For this review, take the finished solid that the model builds, in its own axes (mm). A direction names the side the tool comes from. Give positions to 0.01 mm unless a question says otherwise; leave off trailing zeros. Write each loop counter-clockwise with the first axis right and the second up, starting at its lowest first coordinate (ties: lowest second). Pieces come first, ordered by that corner, then holes. Notation, with made-up numbers: (-24, 50.5) -> (-15, 50.5) arc R20 cw to (-15, 58.5) -> close; hole circle Ø7 at (89, 53.5). An arc over 180 degrees is marked (long way). Return JSON: item names as keys, results as strings.
Autodesk Fusion 360 part; units mm, degrees
sketch "Sketch1" plane through (0, 0, 0) normal (0, 0, 1) x (1, 0, 0)
  line L0 (36.9, -48.5) -> (-36.9, -48.5)
  line L1 (-36.9, -48.5) -> (-36.9, 48.5)
  line L2 (-36.9, 48.5) -> (36.9, 48.5)
  line L3 (36.9, 48.5) -> (36.9, -48.5)
  line L4 (36.9, -48.5) -> (-36.9, 48.5) construction
  line L5 (-36.9, -48.5) -> (36.9, 48.5) construction
  line L6 (35.35, -46.95) -> (-35.35, -46.95)
  line L7 (-35.35, -46.95) -> (-35.35, 46.95)
  line L8 (-35.35, 46.95) -> (35.35, 46.95)
  line L9 (35.35, 46.95) -> (35.35, -46.95)
  line L10 (35.35, -46.95) -> (-35.35, 46.95) construction
  line L11 (-35.35, -46.95) -> (35.35, 46.95) construction
  line L12 (35.35, -46.95) -> (0, -46.95)
  line L13 (0, -46.95) -> (0, -16.95)
  line L14 (11.5, -10.35) -> (-11.5, -10.35)
  line L15 (-11.5, -10.35) -> (-11.5, -23.55)
  line L16 (-11.5, -23.55) -> (11.5, -23.55)
  line L17 (11.5, -23.55) -> (11.5, -10.35)
  line L18 (11.5, -10.35) -> (-11.5, -23.55) construction
  line L19 (-11.5, -10.35) -> (11.5, -23.55) construction
  line L20 (13.775, -30.9) -> (-13.775, -30.9)
  line L21 (-13.775, -30.9) -> (-13.775, -3)
  line L22 (-13.775, -3) -> (13.775, -3)
  line L23 (13.775, -3) -> (13.775, -30.9)
  line L24 (13.775, -30.9) -> (-13.775, -3) construction
  line L25 (-13.775, -30.9) -> (13.775, -3) construction
  line L26 (13.775, -3) -> (11.975, -3)
  line L27 (-13.775, -3) -> (-11.975, -3)
  line L28 (-13.775, -30.9) -> (-11.975, -30.9)
  line L29 (13.775, -30.9) -> (11.975, -30.9)
  line L30 (-11.975, -30.9) -> (-13.775, -30.9)
  line L31 (-13.775, -30.9) -> (-13.775, -29.1)
  line L32 (-13.775, -29.1) -> (-11.975, -29.1)
  line L33 (-11.975, -29.1) -> (-11.975, -30.9)
  line L34 (11.975, -30.9) -> (13.775, -30.9)
  line L35 (13.775, -30.9) -> (13.775, -29.1)
  line L36 (13.775, -29.1) -> (11.975, -29.1)
  line L37 (11.975, -29.1) -> (11.975, -30.9)
  line L38 (-11.975, -3) -> (-13.775, -3)
  line L39 (-13.775, -3) -> (-13.775, -4.8)
  line L40 (-13.775, -4.8) -> (-11.975, -4.8)
  line L41 (-11.975, -4.8) -> (-11.975, -3)
  line L42 (11.975, -3) -> (13.775, -3)
  line L43 (13.775, -3) -> (13.775, -4.8)
  line L44 (13.775, -4.8) -> (11.975, -4.8)
  line L45 (11.975, -4.8) -> (11.975, -3)
  circle A0 centre (-11.975, -4.8) radius 1.1
  circle A1 centre (11.975, -4.8) radius 1.1
  circle A2 centre (11.975, -29.1) radius 1.1
  circle A3 centre (-11.975, -29.1) radius 1.1
  circle A4 centre (-25, 20) radius 2.45
  point P0 (0, -16.95)
  point P1 (0, -16.95)
  dimension "d1" = 73.8
  dimension "d2" = 97
  dimension "d3" = 70.7
  dimension "d4" = 93.9
  dimension "d48" = 30
  dimension "d49" = 23
  dimension "d50" = 13.2
  dimension "d51" = 27.55
  dimension "d52" = 27.9
  dimension "d53" = 1.8
  dimension "d54" = 1.8
  dimension "d55" = 1.8
  dimension "d56" = 1.8
  dimension "d57" = 1.8
  dimension "d58" = 1.8
  dimension "d59" = 1.8
  dimension "d60" = 1.8
  dimension "d61" = 2.2
  dimension "d62" = 2.2
  dimension "d63" = 2.2
  dimension "d64" = 2.2
  dimension "d67" = 4.9
extrude "Extrude1" add sketch "Sketch1" along normal blind 2.5 contours L0 L1 L2 L3 | L14 L15 L16 L17 | L20 L21 L22 L23 L32 L33 L36 L37 L40 L41 L44 L45 A0 A1 A2 A3 | L6 L7 L8 L9 L12 | L20 L23 L29 L34 L35 L36 L37 A2 | L20 L21 L28 L30 L31 L32 L33 A3 | L36 L37 A2 | L36 L37 A2 | L32 L33 A3 | L32 L33 A3 | L22 L23 L26 L42 L43 L44 L45 A1 | L21 L22 L27 L38 L39 L40 L41 A0 | L44 L45 A1 | L44 L45 A1 | L40 L41 A0 | L40 L41 A0 | A4
extrude "Extrude2" add sketch "Sketch1" along normal blind 12.7 contours L0 L1 L2 L3
fillet "Fillet1" radius 2 8 edges at (-35.35, 46.95, 7.6) (35.35, 46.95, 7.6) (35.35, -46.95, 7.6) (-35.35, -46.95, 7.6) (-36.9, -48.5, 6.35) (36.9, -48.5, 6.35) (36.9, 48.5, 6.35) (-36.9, 48.5, 6.35)
fillet "Fillet2" radius 1 8 edges at (-36.3142, -47.9142, 0) (0, -48.5, 0) (36.3142, -47.9142, 0) (36.9, 0, 0) (36.3142, 47.9142, 0) (0, 48.5, 0) (-36.3142, 47.9142, 0) (-36.9, 0, 0)
sketch "Sketch2" plane through (0, 0, 12.7) normal (0, 0, 1) x (-1, 0, 0)
  line L0 (33.35, -46.95) -> (-33.35, -46.95)
  arc A0 (-35.35, -44.95) -> (-33.35, -46.95) centre (-33.35, -44.95) ccw
  line L1 (-35.35, -44.95) -> (-35.35, 44.95)
  arc A1 (-33.35, 46.95) -> (-35.35, 44.95) centre (-33.35, 44.95) ccw
  line L2 (-33.35, 46.95) -> (33.35, 46.95)
  arc A2 (35.35, 44.95) -> (33.35, 46.95) centre (33.35, 44.95) ccw
  line L3 (35.35, 44.95) -> (35.35, -44.95)
  arc A3 (33.35, -46.95) -> (35.35, -44.95) centre (33.35, -44.95) ccw
  arc A4 (34.9, -48.5) -> (36.9, -46.5) centre (34.9, -46.5) ccw
  line L4 (36.9, -46.5) -> (36.9, 46.5)
  arc A5 (36.9, 46.5) -> (34.9, 48.5) centre (34.9, 46.5) ccw
  line L5 (34.9, 48.5) -> (-34.9, 48.5)
  arc A6 (-34.9, 48.5) -> (-36.9, 46.5) centre (-34.9, 46.5) ccw
  line L6 (-36.9, 46.5) -> (-36.9, -46.5)
  arc A7 (-36.9, -46.5) -> (-34.9, -48.5) centre (-34.9, -46.5) ccw
  line L7 (-34.9, -48.5) -> (34.9, -48.5)
  line L8 (-34.9, 48.5) -> (-34.9, 37.6)
  line L9 (-34.9, 37.6) -> (-35.35, 37.6)
  line L10 (-35.35, 37.6) -> (-36.9, 37.6)
  line L11 (-36.9, 37.6) -> (-36.9, 24.096)
  line L12 (-36.9, 24.096) -> (-35.35, 24.096)
  line L13 (-35.35, 24.096) -> (-35.35, 37.6)
  line L14 (-34.9, 48.5) -> (-34.9, -48.5)
  line L15 (-34.9, -48.5) -> (-34.9, -37.6)
  line L16 (-34.9, -37.6) -> (-34.9, -24.096)
  line L17 (-34.9, -24.096) -> (-36.4, -24.096)
  line L18 (-36.9, -23.896) -> (-25.5, -23.896)
  line L19 (-25.5, -23.896) -> (-25.5, -37.4)
  line L20 (-25.5, -37.4) -> (-36.9, -37.4)
  line L21 (-36.9, -37.4) -> (-36.9, -23.896)
  line L22 (-36.9, -23.896) -> (-36.9, -19.396)
  line L23 (-34.9, -48.5) -> (-34.9, -37.6)
  line L24 (-34.9, -37.6) -> (-36.9, -37.5994)
  dimension "d13" = 10.9
  dimension "d14" = 13.504
  dimension "d19" = 10.9
  dimension "d20" = 13.504
  dimension "d21" = 1.5
  dimension "d22" = 13.504
  dimension "d31" = 4.5
  dimension "d47" = 10.9
extrude "Extrude5" cut sketch "Sketch2" against normal blind 9.5 contours L1 L14 L16 L17 L20 | L1 L6 L18 L20 L21
fillet "Fillet5" radius 3 2 edges at (36.125, 23.896, 3.2) (36.125, 37.4, 3.2)
sketch "Sketch3" plane through (36.9, 0, 0) normal (1, 0, 0) x (0, 1, 0)
  line L0 (37.4, 12.7) -> (37.4, 6.2)
  arc A0 (34.4, 3.2) -> (37.4, 6.2) centre (34.4, 6.2) ccw
  line L1 (34.4, 3.2) -> (26.896, 3.2)
  arc A1 (23.896, 6.2) -> (26.896, 3.2) centre (26.896, 6.2) ccw
  line L2 (23.896, 6.2) -> (23.896, 12.7)
  line L3 (23.896, 12.7) -> (-46.5, 12.7)
  line L4 (-46.5, 12.7) -> (-46.5, 1)
  line L5 (-46.5, 1) -> (46.5, 1)
  line L6 (46.5, 1) -> (46.5, 12.7)
  line L7 (46.5, 12.7) -> (37.4, 12.7)
  line L8 (23.896, 12.7) -> (19.396, 12.7)
  line L9 (19.396, 12.7) -> (19.396, 2.68)
  line L10 (19.396, 12.7) -> (19.396, 10.19)
  line L11 (19.396, 10.19) -> (7.307, 10.19)
  line L12 (7.307, 10.19) -> (7.307, 5.19)
  line L13 (7.307, 5.19) -> (19.396, 5.19)
  line L14 (19.396, 5.19) -> (19.396, 10.19)
  dimension "d32" = 4.5
  dimension "d33" = 10.02
  dimension "d34" = 2.51
  dimension "d35" = 12.089
  dimension "d36" = 5
extrude "Extrude6" cut sketch "Sketch3" against normal blind 2 contours L9 L11 L12 L13 L14
fillet "Fillet6" radius 2.5 4 edges at (36.125, 7.307, 10.19) (36.125, 19.396, 10.19) (36.125, 19.396, 5.19) (36.125, 7.307, 5.19)
sketch "Sketch4" plane through (-35.35, 0, 0) normal (1, 0, 0) x (0, 1, 0)
  line L0 (-44.95, 12.7) -> (-44.95, 2.5)
  line L1 (-44.95, 2.5) -> (44.95, 2.5)
  line L2 (44.95, 2.5) -> (44.95, 12.7)
  line L3 (44.95, 12.7) -> (-44.95, 12.7)
  line L4 (44.95, 12.7) -> (30.837, 12.7)
  line L5 (30.837, 12.7) -> (30.837, 7.306)
  line L6 (30.837, 12.7) -> (30.837, 2.5)
  line L7 (30.837, 2.5) -> (30.837, 13.991)
  circle A0 centre (30.837, 13.991) radius 6.1
  line L8 (36.7988, 12.7) -> (44.95, 12.7)
  dimension "d41" = 14.113
  dimension "d42" = 5.394
  dimension "d43" = 11.491
  dimension "d44" = 12.2
extrude "Extrude7" cut sketch "Sketch4" against normal blind 2 contours L3 L5 L6 L7 A0 | L3 L4 L5 L6 L7 A0
extrude "Extrude8" cut sketch "Sketch1" along normal blind 4 contours L14 L15 L16 L17 | L36 L37 A2 | L36 L37 A2 | L32 L33 A3 | L32 L33 A3 | L44 L45 A1 | L44 L45 A1 | L40 L41 A0 | L40 L41 A0
extrude "Extrude9" cut sketch "Sketch1" along normal blind 5 contours A4
1. The part is to be moulded in two halves that separate along X. For faces 1 (the flat face through (36.9, 1, 7)), 2 (the cylindrical face through (-36.33, 47.9, 6.77)), 3 (the flat face through (11.5, -17, 1)), 4 (the flat face through (-1, 1, 0)), say which applies: +X half, -X half, draft (parallel to the pull), parting line (faces both ways), or undercut.
Results found:
{"face 1": "+X half", "face 2": "-X half", "face 3": "undercut", "face 4": "draft"}
2. To check wall thickness, follow probe 1 along Y at (x, z) = (17, 8.75); probe 2 along X at (y, z) = (38, 10); probe 3 along X at (y, z) = (-11, 1.5). State the ranges of each line that lie inside material, in increasing order.
Results found:
{"probe 1": "y = -48.5 to -46.95, 46.95 to 48.5", "probe 2": "x = -36.9 to -35.35, 35.35 to 36.9", "probe 3": "x = -36.9 to -11.5, 11.5 to 36.9"}
3. Add section D-D, the plane x = 18. State the section outline as (y, z) points.
Results found:
{"outline": "(-48.5, 1) arc R1 ccw to (-47.5, 0) -> (47.5, 0) arc R1 ccw to (48.5, 1) -> (48.5, 12.7) -> (46.95, 12.7) -> (46.95, 2.5) -> (-46.95, 2.5) -> (-46.95, 12.7) -> (-48.5, 12.7) -> close"}
4. For pin 1 (1.7 mm diameter, centred on x = 36.5, y = 31.5, fed in from +Z); pin 2 (8 mm diameter, centred on x = -25, y = 20, fed in from +Z); pin 3 (2 mm diameter, centred on x = -11.975, y = -4.8, fed in from -Z), all flat-tipped, find the tip position at first contact; note any pin that passes through.
Results found:
{"pin 1": "stops at z = 3.2", "pin 2": "stops at z = 2.5", "pin 3": "passes through"}
5. For faces 5 (the cylindrical face through (36.11, 8.06, 5.9)), 6 (the flat face through (-11.5, -17, 1)), 7 (the flat face through (0, 46.95, 8)), 8 (the cylindrical face through (36.114, 24.798, 4.055)), list the 3-axis set-ups (+Z, -Z, +X, -X, +Y, -Y) from which the entire face can be reached by the end or side of a thin tool; tool diameter is ignored.
Results found:
{"face 5": "+X", "face 6": "+Z, -Z", "face 7": "+Z", "face 8": "+Z, +X"}
6. Add section A-A, the plane x = -25. State the section outline as (y, z) points.
Results found:
{"outline": "(-48.5, 1) arc R1 ccw to (-47.5, 0) -> (17.55, 0) -> (17.55, 2.5) -> (-46.95, 2.5) -> (-46.95, 12.7) -> (-48.5, 12.7) -> close; (22.45, 0) -> (47.5, 0) arc R1 ccw to (48.5, 1) -> (48.5, 12.7) -> (46.95, 12.7) -> (46.95, 2.5) -> (22.45, 2.5) -> close"}
7. Add section B-B, the plane y = -4.8. State the section outline as (x, z) points (3 decimals), plus the area to 3 significant figures.
Results found:
{"outline": "(-36.9, 1) arc R1 ccw to (-35.9, 0) -> (-13.075, 0) -> (-13.075, 2.5) -> (-35.35, 2.5) -> (-35.35, 12.7) -> (-36.9, 12.7) -> close; (-10.875, 0) -> (10.875, 0) -> (10.875, 2.5) -> (-10.875, 2.5) -> close; (13.075, 0) -> (35.9, 0) arc R1 ccw to (36.9, 1) -> (36.9, 12.7) -> (35.35, 12.7) -> (35.35, 2.5) -> (13.075, 2.5) -> close", "area": "205 mm²"}
8. Add section C-C, the plane y = -18. State the section outline as (x, z) points, plus the area to 3 significant figures.
Results found:
{"outline": "(-36.9, 1) arc R1 ccw to (-35.9, 0) -> (-11.5, 0) -> (-11.5, 2.5) -> (-35.35, 2.5) -> (-35.35, 12.7) -> (-36.9, 12.7) -> close; (11.5, 0) -> (35.9, 0) arc R1 ccw to (36.9, 1) -> (36.9, 12.7) -> (35.35, 12.7) -> (35.35, 2.5) -> (11.5, 2.5) -> close", "area": "158 mm²"}
